from build123d import *
from build123d.topology import SkipClean

# Parameters (mm, degrees)
SKETCH1_R           = 10
BOSS_EXTRUDE1_DEPTH = 15.7
SKETCH2_R           = 3
BOSS_EXTRUDE2_DEPTH = 1.3
BOSS_EXTRUDE3_DEPTH = 0.8
FILLET1_R           = 2
SKETCH4_R           = 2.5
BOSS_EXTRUDE4_DEPTH = 1.3
SKETCH5_R           = 0.75
BOSS_EXTRUDE5_DEPTH = 9.7
BOSS_EXTRUDE6_START = 1.2
SKETCH6_R           = 0.75
BOSS_EXTRUDE6_DEPTH = 1.2


with BuildPart() as part:
    # Sketch1 → Boss-Extrude1 (new body)
    with BuildSketch(Plane(origin=(0, 0, 0), x_dir=(1, 0, 0), z_dir=(0, 1, 0))):
        with Locations(Location((0, 0, 0), (0, 0, 270))):
            Circle(SKETCH1_R)
    extrude(amount=BOSS_EXTRUDE1_DEPTH)

    # Sketch2 → Boss-Extrude2 (add)
    with BuildSketch(Plane.XZ):
        with Locations(Location((0, 0, 0), (0, 0, 90))):
            Circle(SKETCH2_R)
    extrude(amount=BOSS_EXTRUDE2_DEPTH)

    # Sketch3 → Boss-Extrude3 (add)
    with SkipClean():  # the faces are left unmerged after this step: merging them gives an invalid solid
        with BuildSketch(Plane(origin=(0, 15.7, 0), x_dir=(1, 0, 0), z_dir=(0, 1, 0))):
            with BuildLine():
                Line((-14.671400751, 5), (-3.642056653, 9.313185456))
                ThreePointArc((-3.642056653, 9.313185456), (0, 10), (3.642056653, 9.313185456))
                Line((3.642056653, 9.313185456), (14.671400751, 5))
                ThreePointArc((14.671400751, 5), (15.5, 0), (14.671400751, -5))
                Line((14.671400751, -5), (3.642056653, -9.313185456))
                ThreePointArc((3.642056653, -9.313185456), (0, -10), (-3.642056653, -9.313185456))
                Line((-3.642056653, -9.313185456), (-14.671400751, -5))
                ThreePointArc((-14.671400751, -5), (-15.5, 0), (-14.671400751, 5))
            make_face()
            with BuildLine():
                ThreePointArc((-13.442625829, 2.370297625), (-13.65, 0), (-13.442625829, -2.370297625))
                ThreePointArc((-13.442625829, -2.370297625), (-12.110401508, -3.303131137), (-11.177567997, -1.970906817))
                ThreePointArc((-11.177567997, -1.970906817), (-11.35, 0), (-11.177567997, 1.970906817))
                ThreePointArc((-11.177567997, 1.970906817), (-12.110401508, 3.303131137), (-13.442625829, 2.370297625))
            make_face(mode=Mode.SUBTRACT)
            with BuildLine():
                ThreePointArc((13.442625829, -2.370297625), (13.65, 0), (13.442625829, 2.370297625))
                ThreePointArc((13.442625829, 2.370297625), (12.110401508, 3.303131137), (11.177567997, 1.970906817))
                ThreePointArc((11.177567997, 1.970906817), (11.35, 0), (11.177567997, -1.970906817))
                ThreePointArc((11.177567997, -1.970906817), (12.110401508, -3.303131137), (13.442625829, -2.370297625))
            make_face(mode=Mode.SUBTRACT)
        extrude(amount=BOSS_EXTRUDE3_DEPTH)

    # Fillet1
    fillet1_edges = [part.edges().sort_by_distance(p)[0] for p in [
        (-14.671400751, 16.1, -5),
        (14.671400751, 16.1, -5),
        (14.671400751, 16.1, 5),
        (-14.671400751, 16.1, 5),
    ]]
    fillet(fillet1_edges, radius=FILLET1_R)

    # Sketch4 → Boss-Extrude4 (add)
    with SkipClean():  # the faces are left unmerged after this step: merging them gives an invalid solid
        with BuildSketch(Plane(origin=(0, 16.5, 0), x_dir=(1, 0, 0), z_dir=(0, 1, 0))):
            with Locations(Location((0, 0, 0), (0, 0, 270))):
                Circle(SKETCH4_R)
        extrude(amount=BOSS_EXTRUDE4_DEPTH)

    # Sketch5 → Boss-Extrude5 (add)
    with SkipClean():  # the faces are left unmerged after this step: merging them gives an invalid solid
        with BuildSketch(Plane(origin=(0, 17.8, 0), x_dir=(1, 0, 0), z_dir=(0, 1, 0))):
            with Locations(Location((0, 0, 0), (0, 0, 270))):
                Circle(SKETCH5_R)
        extrude(amount=BOSS_EXTRUDE5_DEPTH)

    # Sketch6 → Boss-Extrude6 (add)
    with SkipClean():  # the faces are left unmerged after this step: merging them gives an invalid solid
        with BuildSketch(Plane.XZ.offset(1.3).offset(BOSS_EXTRUDE6_START)):
            with Locations(Location((0, 0, 0), (0, 0, 90))):
                Circle(SKETCH6_R)
        extrude(amount=-BOSS_EXTRUDE6_DEPTH)


solid = part.part
Could you check a few things on this model? Use its own coordinates, in mm. A direction names the side the tool comes from. Give positions to 0.01 mm unless a question says otherwise; leave off trailing zeros. Order: outer loops, then holes, each group sorted by start corner. A loop starts at its lowest first (then second) coordinate and runs counter-clockwise, first axis right, second up. Notation, with made-up numbers: (6, 29) -> (46, 29) arc R17 ccw to (46, 39) -> close; hole circle Ø3 at (-38, 88.5). An arc over 180 degrees is marked (long way). Return JSON: item names as keys, results as strings.
1. For pin 1 Ø1 at (x, z) = (-9, -7.5) entering from -Y; pin 2 Ø3 at (y, z) = (11.5, 6.5) entering from -X; pin 3 Ø3.5 at (x, z) = (-7, 3.5) entering from -Y; pin 4 Ø1.5 at (x, z) = (-0.5, -1) entering from +Y, each with a flat end and sliding along its axis, tell me the tip position at first contact or that it passes through.
Answer list:
{"pin 1": "stops at y = 15.7", "pin 2": "stops at x = -8.66", "pin 3": "stops at y = 0", "pin 4": "stops at y = 27.5"}
2. Imagine slicing it at C-C on y = 13.25. List the corners of the cut face in (x, z) for me, then the cut area to 3 significant figures.
Answer list:
{"outline": "circle Ø20 at (0, 0)", "area": "314 mm2"}
3. Thinking about a two-plate mould opening in X: for faces 4 (the cylindrical face through (-15.5, 16.1, 0.1)), 5 (the flat face through (0, -2.5, 0)), 6 (the cylindrical face through (13.65, 16.09, 0.03)), which applies, pulls with the +X half, pulls with the -X half, needs draft (parallel to the pull), parting line crosses it, or undercut?
Answer list:
{"face 4": "pulls with the -X half", "face 5": "needs draft", "face 6": "undercut"}
4. Imagine slicing it at A-A on z = 0. Give the number of separate pieces and of enclosed holes in the cut face, then the cut area to 3 significant figures.
Answer list:
{"separate pieces": "3", "enclosed holes": "0", "area": "366 mm2"}
5. I need wall thicknesses on line 1 (Y direction, x = -0.5, z = 5.5); line 2 (X direction, y = 4, z = 4); line 3 (X direction, y = 3.25, z = 0). Which ranges of each line are inside material? Lowest first, please. Write a range as from..to.
Answer list:
{"line 1": "y = 0..16.5", "line 2": "x = -9.17..9.17", "line 3": "x = -10..10"}
6. Imagine slicing it at B-B on x = 0. List the corners of the cut face in (y, z) for me.
Answer list:
{"outline": "(-2.5, -0.75) -> (-1.3, -0.75) -> (-1.3, -3) -> (0, -3) -> (0, -10) -> (16.5, -10) -> (16.5, -2.5) -> (17.8, -2.5) -> (17.8, -0.75) -> (27.5, -0.75) -> (27.5, 0.75) -> (17.8, 0.75) -> (17.8, 2.5) -> (16.5, 2.5) -> (16.5, 10) -> (0, 10) -> (0, 3) -> (-1.3, 3) -> (-1.3, 0.75) -> (-2.5, 0.75) -> close"}
7. Imagine slicing it at D-D on z = 5.75. List the corners of the cut face in (x, y) for me.
Answer list:
{"outline": "(-12.75, 15.7) -> (-8.18, 15.7) -> (-8.18, 0) -> (8.18, 0) -> (8.18, 15.7) -> (12.75, 15.7) -> (12.75, 16.5) -> (-12.75, 16.5) -> close"}
8. On a 3-axis mill with a long thin cutter (end or side, diameter ignored), from which of +Z, -Z, +X, -X, +Y, -Y can I reach the whole of each face in a straight line? I mean faces 1 (the flat face through (1, 17.8, 1)), 2 (the flat face through (-11, 15.7, -1)), 3 (the cylindrical face through (-11.35, 16.09, 0.03)). Say none if no direction works.
Answer list:
{"face 1": "+Y", "face 2": "-X, -Y", "face 3": "+Y, -Y"}
